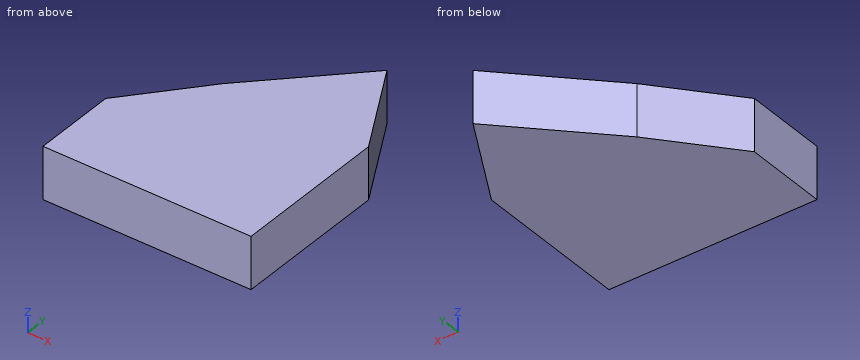
from build123d import *

# Parameters (mm, degrees)
F0_W     = 100
F0_H     = 20
F1_DEPTH = 25


with BuildPart() as f1:
    # F0 (on Top) → F1 (new body)
    with BuildSketch(Plane.XY):
        Polygon((1.057282, 131.128362), (-43.942718, 86.128362), (26.057282, 86.128362), align=None)
        Polygon((-43.942718, 86.128362), (-73.942718, 51.128362), (26.057282, 51.128362), (26.057282, 86.128362), align=None)
        with Locations((-23.942718, 41.128362)):
            Rectangle(F0_W, F0_H)
        with Locations((-23.942718, 21.128362)):
            Rectangle(F0_W, F0_H)
    extrude(amount=F1_DEPTH)


solid = f1.part
Read the model definition and answer for the solid it produces. Units are mm, in the model's axes. Give positions to 0.01 mm unless a question says otherwise; leave off trailing zeros. Write each loop counter-clockwise with the first axis right and the second up, starting at its lowest first coordinate (ties: lowest second). Pieces come first, ordered by that corner, then holes. Notation, with made-up numbers: (89, -11.5) - (125, -11.5) arc R10 ccw to (125, 0.5) - close; hole circle Ø1 at (18, 46). An arc over 180 degrees is marked (long way). Answer in a Markdown table with one row per item. Add a question column.
Item 1: Section C-C, the plane x = 13 is taken. Write down the section's boundary in (y, z), and give its area (3 significant figures).
Item 2: Section A-A, the plane z = 14 is taken. Write down the section's boundary in (x, y), and give its area (3 significant figures).
Item 3: Section B-B, the plane y = 117 is taken. Write down the section's boundary in (x, z), and give its area (3 significant figures).
Item 4: A flat-ended cylindrical pin translates along its axis: P1, Ø12, axis at y = 103, z = 11.5, coming from the +X side. Find the tip coordinate at first contact, or state that the pin passes through.
Item 5: Find the intervals of material crossed by L1, parallel to X at y = 123.5, z = 6.25; L2, parallel to Y at x = -13, z = 12; L3, parallel to Y at x = 4, z = 15.75, in increasing order.
Recorded:
| question | item | result |
|---|---|---|
| 1 | outline | (11.13, 0) - (109.63, 0) - (109.63, 25) - (11.13, 25) - close |
| 1 | area | 2,460 mm2 |
| 2 | outline | (-73.94, 11.13) - (26.06, 11.13) - (26.06, 86.13) - (1.06, 131.13) - (-43.94, 86.13) - (-73.94, 51.13) - close |
| 2 | area | 8,550 mm2 |
| 3 | outline | (-13.07, 0) - (8.91, 0) - (8.91, 25) - (-13.07, 25) - close |
| 3 | area | 549 mm2 |
| 4 | P1 | stops at x = 20.02 |
| 5 | L1 | x = -6.57 to 5.3 |
| 5 | L2 | y = 11.13 to 117.07 |
| 5 | L3 | y = 11.13 to 125.83 |
